```python
from build123d import *

# Parameters (mm, degrees)
CROQUIS1_R              = 3.65
CROQUIS1_R_2            = 2.65
SALIENTE_EXTRUIR1_DEPTH = 3.5
CROQUIS2_R              = 3.65
SALIENTE_EXTRUIR2_DEPTH = 3.5
CROQUIS3_R              = 2.15
SALIENTE_EXTRUIR3_DEPTH = 3.5


with BuildPart() as part:
    # Croquis1 → Saliente-Extruir1 (new body)
    with BuildSketch(Plane(origin=(0, 0, 0), x_dir=(1, 0, 0), z_dir=(0, 1, 0))):
        Circle(CROQUIS1_R)
        Circle(CROQUIS1_R_2, mode=Mode.SUBTRACT)
    extrude(amount=SALIENTE_EXTRUIR1_DEPTH)

    # Croquis2 → Saliente-Extruir2 (add)
    with BuildSketch(Plane(origin=(0, 3.5, 0), x_dir=(1, 0, 0), z_dir=(0, 1, 0))):
        Circle(CROQUIS2_R)
    extrude(amount=SALIENTE_EXTRUIR2_DEPTH)

    # Croquis3 → Saliente-Extruir3 (add)
    with BuildSketch(Plane(origin=(0, 7, 0), x_dir=(1, 0, 0), z_dir=(0, 1, 0))):
        Circle(CROQUIS3_R)
    extrude(amount=SALIENTE_EXTRUIR3_DEPTH)


solid = part.part
```
Part model, mm, in its own coordinate system. A direction names the side the tool comes from. Coordinates: 2 decimals unless noted, no trailing zeros. Loops run counter-clockwise (first coordinate to the right, second up) from the corner with the lowest first, then second, coordinate; pieces in that order, holes last. Notation, with made-up numbers: (-20.5, 10) - (21.5, 10) arc R25 cw to (21.5, 47) - close; hole circle Ø9 at (24.25, 54). An arc over 180 degrees is marked (long way). Write item = value, one per line. Start each with the question number.
Item 1: 3-axis set-ups, long thin cutter, end or side, ignore diameter. For faces 1 (the cylindrical face through (2.45, 1.73, 1.01)), 2 (the cylindrical face through (-2.15, 8.73, -0.09)), 3 (the flat face through (2, 0, -2)): which of +Z, -Z, +X, -X, +Y, -Y reach the whole face in a straight line?
Item 2: Wall check: L1, parallel to Z at x = 0, y = 2.05; L2, parallel to Y at x = -0.5, z = 1. Give the ranges that are in metal, low to high. Write a range as from..to.
Item 3: Flat gauge pin, fed straight in: pin 1 Ø2 at (x, y) = (1.5, 9.5) entering from +Z. Where does the tip first touch, or does it go through?
Item 4: Mould opens along Z. For faces 4 (the flat face through (0, 3.5, 0)), 5 (the cylindrical face through (3.48, 3.45, -1.1)), 6 (the flat face through (2, 7, 2)) say: released by +Z, released by -Z, zero draft, split by the parting line, or undercut.
Item 5: Cut at A-A, the plane x = 0. Give the cut face in (y, z).
Item 6: Cut at C-C, the plane y = 5.5. Give the cut face in (x, z).
Item 7: Cut at D-D, the plane y = 0.5. Give the cut face in (x, z).
Item 8: Cut at B-B, the plane z = 0. Give the cut face in (x, y), and give its area (3 significant figures).
The answers:
q1.face_1 = -Y
q1.face_2 = +Y
q1.face_3 = +Z, -Z, +X, -X, -Y
q2.L1 = -3.65..-2.65, 2.65..3.65
q2.L2 = 3.5..10.5
q3.pin_1 = 2.09
q4.face_4 = undercut
q4.face_5 = split by the parting line
q4.face_6 = zero draft
q5.outline = (0, -3.65) - (7, -3.65) - (7, -2.15) - (10.5, -2.15) - (10.5, 2.15) - (7, 2.15) - (7, 3.65) - (0, 3.65) - (0, 2.65) - (3.5, 2.65) - (3.5, -2.65) - (0, -2.65) - close
q6.outline = circle Ø7.3 at (0, 0)
q7.outline = circle Ø7.3 at (0, 0); hole circle Ø5.3 at (0, 0)
q8.outline = (-3.65, 0) - (-2.65, 0) - (-2.65, 3.5) - (2.65, 3.5) - (2.65, 0) - (3.65, 0) - (3.65, 7) - (2.15, 7) - (2.15, 10.5) - (-2.15, 10.5) - (-2.15, 7) - (-3.65, 7) - close
q8.area = 47.6 mm2
